```python
from build123d import *

# Parameters (mm, degrees)
EXTRUDE_THIN1_DEPTH = 533.4
FILLET1_R           = 1.27


with BuildPart() as part:
    # Sketch1 → Extrude-Thin1 (new body)
    with BuildSketch(Plane.XY):
        with BuildLine():
            Line((0, 0), (-3.175, 0))
            ThreePointArc((-3.175, 0), (-6.294965924, 8.894339761), (-14.2875, 13.890625))
            Line((-14.2875, 13.890625), (-14.2875, 18.653125))
            Line((-14.2875, 18.653125), (-17.4625, 18.653125))
            Line((-17.4625, 18.653125), (-17.4625, 47.228125))
            Line((-17.4625, 47.228125), (-14.2875, 47.228125))
            Line((-14.2875, 47.228125), (-14.2875, 51.990625))
            ThreePointArc((-14.2875, 51.990625), (-6.294965924, 56.986910239), (-3.175, 65.88125))
            Line((-3.175, 65.88125), (0, 65.88125))
            Line((0, 65.88125), (0, 64.61125))
            Line((0, 64.61125), (-1.957090043, 64.61125))
            ThreePointArc((-1.957090043, 64.61125), (-5.380817599, 56.097391338), (-13.0175, 51.009289373))
            Line((-13.0175, 51.009289373), (-13.0175, 45.958125))
            Line((-13.0175, 45.958125), (-16.1925, 45.958125))
            Line((-16.1925, 45.958125), (-16.1925, 19.923125))
            Line((-16.1925, 19.923125), (-13.0175, 19.923125))
            Line((-13.0175, 19.923125), (-13.0175, 14.871960627))
            ThreePointArc((-13.0175, 14.871960627), (-5.380817599, 9.783858662), (-1.957090043, 1.27))
            Line((-1.957090043, 1.27), (0, 1.27))
            Line((0, 1.27), (0, 0))
        make_face()
    extrude(amount=-EXTRUDE_THIN1_DEPTH)

    # Fillet1
    fillet1_edges = [part.edges().sort_by_distance(p)[0] for p in [
        (-3.175, 0, -266.7),
        (-14.2875, 13.890625, -266.7),
        (-17.4625, 18.653125, -266.7),
        (-17.4625, 47.228125, -266.7),
        (-14.2875, 51.990625, -266.7),
        (-3.175, 65.88125, -266.7),
        (-13.0175, 45.958125, -266.7),
        (-13.0175, 19.923125, -266.7),
    ]]
    fillet(fillet1_edges, radius=FILLET1_R)


solid = part.part
```
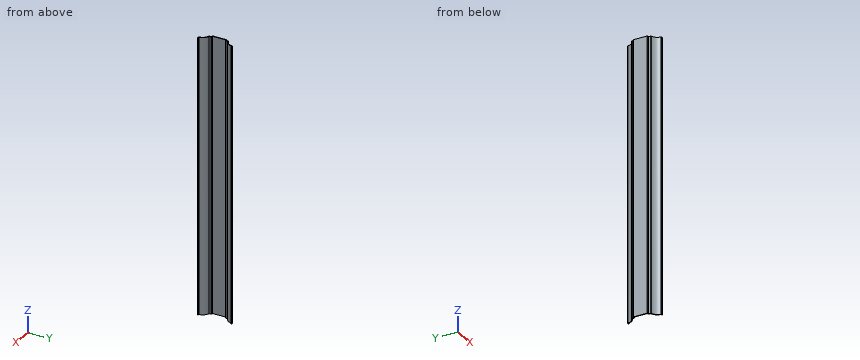
Build history of the part. All positions in model axes, mm. Round coordinates to 2 decimals unless told otherwise and drop trailing zeros. Write each loop counter-clockwise with the first axis right and the second up, starting at its lowest first coordinate (ties: lowest second). Pieces come first, ordered by that corner, then holes.
1) Band-saw the part on B-B, the plane z = -166.5. List the corners of the cut face in (x, y).
2) Pin check, flat tips, straight feed: pin 1 (2 mm diameter, centred on x = -12, z = -109, fed in from -Y); pin 2 (4 mm diameter, centred on y = 49.5, z = -250, fed in from -X); pin 3 (2 mm diameter, centred on x = -4, z = -143, fed in from +Y). Stop position of each tip, or through.
3) Drill centre lines: probe 1 along Y at (x, z) = (-1.25, -445); probe 2 along Y at (x, z) = (-15, -80); probe 3 along X at (y, z) = (30, -395). Where is each one in solid material? Low to high.
4) Band-saw the part on A-A, the plane x = -8.75. List the corners of the cut face in (y, z), and give its area (3 significant figures).
5) Band-saw the part on C-C, the plane y = 33. List the corners of the cut face in (x, z).
Ans:
1. outline: (-17.46, 19.92) arc R1.27 ccw to (-16.19, 18.65) - (-14.29, 18.65) - (-14.29, 14.87) arc R1.27 ccw to (-13.38, 13.65) arc R14.24 cw to (-3.22, 1.17) arc R1.27 ccw to (-1.96, 0) - (0, 0) - (0, 1.27) - (-1.96, 1.27) arc R15.51 ccw to (-13.02, 14.87) - (-13.02, 18.65) arc R1.27 ccw to (-14.29, 19.92) - (-16.19, 19.92) - (-16.19, 45.96) - (-14.29, 45.96) arc R1.27 ccw to (-13.02, 47.23) - (-13.02, 51.01) arc R15.51 ccw to (-1.96, 64.61) - (0, 64.61) - (0, 65.88) - (-1.96, 65.88) arc R1.27 ccw to (-3.22, 64.72) arc R14.24 cw to (-13.38, 52.23) arc R1.27 ccw to (-14.29, 51.01) - (-14.29, 47.23) - (-16.19, 47.23) arc R1.27 ccw to (-17.46, 45.96) - close
2. pin 1: stops at y = 12.71
2. pin 2: stops at x = -14.29
2. pin 3: stops at y = 65.34
3. probe 1: y = 0 to 1.27, 64.61 to 65.88
3. probe 2: y = 18.65 to 19.92, 45.96 to 47.23
3. probe 3: x = -17.46 to -16.19
4. outline: (11.3, -533.4) - (12.86, -533.4) - (12.86, 0) - (11.3, 0) - close; (53.02, -533.4) - (54.58, -533.4) - (54.58, 0) - (53.02, 0) - close
4. area: 1,670 mm2
5. outline: (-17.46, -533.4) - (-16.19, -533.4) - (-16.19, 0) - (-17.46, 0) - close
